Answer from the drawing. Dimensions are ordinates in mm from the lowest x, y and z of the part. A direction names the side the tool comes from. Round coordinates to 2 decimals unless told otherwise and drop trailing zeros. Order: outer loops, then holes, each group sorted by start corner. A loop starts at its lowest first (then second) coordinate and runs counter-clockwise, first axis right, second up.
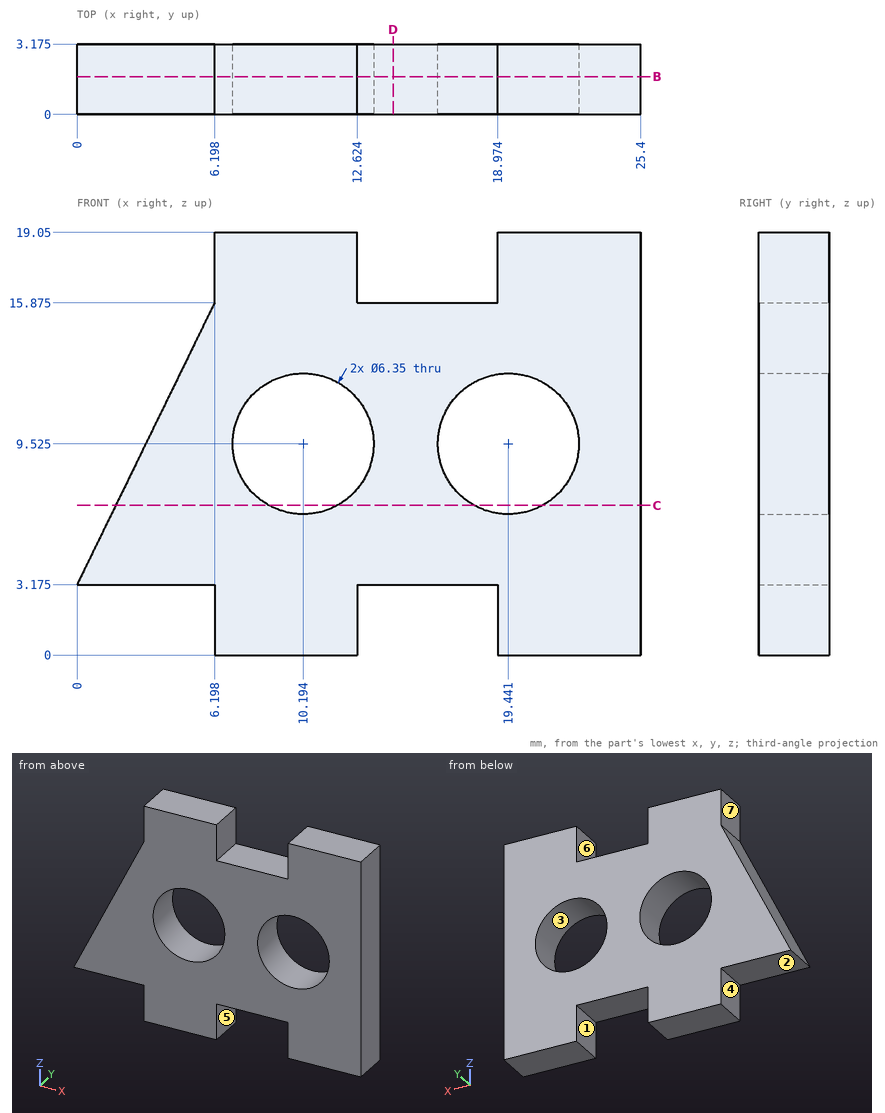
Q1. A cutting plane is placed at D-D, the plane x = 14.25. Give the vertices of the cut face in (y, z) (1 decimal).
Outcome:
outline: (0, 3.2) - (3.2, 3.2) - (3.2, 15.9) - (0, 15.9) - close
Q2. A flat-ended cylindrical pin translates along its axis: pin 1 (1.6 mm diameter, centred on y = 2, z = 2, fed in from -X). Find the tip coordinate at first contact, or state that the pin passes through.
Outcome:
pin 1: stops at x = 6.2
Q3. A cutting plane is placed at C-C, the plane z = 6.75. Give the vertices of the cut face in (x, y) (1 decimal).
Outcome:
outline: (1.7, 0) - (8.7, 0) - (8.7, 3.2) - (1.7, 3.2) - close; (11.7, 0) - (17.9, 0) - (17.9, 3.2) - (11.7, 3.2) - close; (21, 0) - (25.4, 0) - (25.4, 3.2) - (21, 3.2) - close
Q4. A cutting plane is placed at B-B, the plane y = 1.7. Give the number of separate pieces and of enclosed holes in the cut face.
Outcome:
separate pieces: 1
enclosed holes: 2
Q5. For a pull along X with two mould halves and no side action, classify the marked faces 1, 2, 3 and 4 as released by +X, released by -X, zero draft, split by the parting line, or undercut.
Outcome:
face 1: undercut
face 2: zero draft
face 3: undercut
face 4: released by -X
Q6. For the marked faces 5, 6 and 7, determine the directions among +Z, -Z, +X, -X, +Y, -Y from which every point of the face is accessible in a straight line to the end or side of a thin tool.
Outcome:
face 5: -Z, +Y, -Y
face 6: +Z, +Y, -Y
face 7: +Z, -X, +Y, -Y
Q7. Straight lines are drawn through the part: probe 1 along X at (y, z) = (3, 18); probe 2 along X at (y, z) = (2.9, 8) (1 decimal); probe 3 along X at (y, z) = (0.95, 7.25) (1 decimal). For each, find the intervals that lie inside material, in ascending order.
Outcome:
probe 1: x = 6.2 to 12.62, 18.97 to 25.4
probe 2: x = 2.4 to 7.4, 13 to 16.7, 22.2 to 25.4
probe 3: x = 2 to 8, 12.4 to 17.2, 21.7 to 25.4
